Autodesk Inventor part; units mm, degrees
ref_plane "YZ Plane" through (0, 0, 0) normal (1, 0, 0) x (0, 1, 0)
ref_plane "XZ Plane" through (0, 0, 0) normal (0, 1, 0) x (-1, 0, 0)
ref_plane "XY Plane" through (0, 0, 0) normal (0, 0, 1) x (1, 0, 0)
sketch "Sketch1" plane through (0, 0, 0) normal (0, 1, 0) x (-1, 0, 0)
  line L0 (2.1258, 0) -> (-2.1258, 0) construction
  line L1 (0, 4.2515) -> (0, -4.2515) construction
  line L2 (20, 10) -> (-20, 10)
  line L3 (-20, 10) -> (-20, -10)
  line L4 (-20, -10) -> (20, -10)
  line L5 (20, -10) -> (20, 10)
  point P0 (0, 0)
  point P1 (0, 0)
  dimension "d1" = 20
  dimension "d2" = 20
  dimension "d3" = 20
extrude "Extrusion1" add sketch "Sketch1" along normal blind 7
sketch "Sketch2" plane through (0, 7, 0) normal (0, 1, 0) x (1, 0, 0)
  point P0 (0, 0)
  point P1 (10, 0)
  dimension "d6" = 10
hole "Hole1" at (10, 7, 0) direction (0, -1, 0) diameter 5.5 end through all countersink diameter 10.4 countersink angle 90
ref_plane "Work Plane1" through (0, 5, 0) normal (0, 1, 0) x (1, 0, 0)
sketch "Sketch3" plane through (0, 5, 0) normal (0, 1, 0) x (1, 0, 0)
  circle A0 centre (-8.9944, 0) radius 3
  point P0 (0, 0)
  dimension "d15" = 6
extrude "Extrusion2" cut sketch "Sketch3" against normal blind 1.7
fillet "Fillet1" radius 2 4 edges at (-20, 3.5, 10) (-20, 3.5, -10) (20, 3.5, 10) (20, 3.5, -10)
properties part number "MagnetHolderV1"
CAD build for the part. Positions are in the model's coordinates, mm. A direction names the side the tool comes from. Give positions to 0.01 mm unless a question says otherwise; leave off trailing zeros. Write each loop counter-clockwise with the first axis right and the second up, starting at its lowest first coordinate (ties: lowest second). Pieces come first, ordered by that corner, then holes. Notation, with made-up numbers: M -11.75,55 L 28.25,55 A23 cw 28.25,75 Z; hole C 61.25,-26.5 d3. An arc over 180 degrees is marked long. Put each result on its own line as item: value. Start each with the question number.
(1) Band-saw the part on D-D, the plane y = 4. Write the cut outline in (x, z), and give its area (3 significant figures).
(2) Flat gauge pin, fed straight in: pin 1 Ø12 at (x, z) = (-14.5, -4.5) entering from -Y. Where does the tip first touch, or does it go through?
(3) Band-saw the part on C-C, the plane y = 6.25. Write the cut outline in (x, z).
(4) Which spindle directions (+Z, -Z, +X, -X, +Y, -Y) get a long thin tool onto all of the face, cutting with end or side? Do faces 4 (the face through (-9, 3.3, 0)), 5 (the face through (0, 7, 0)). Say none if no direction does.
(5) Probe L1, parallel to X at y = 3.9, z = 0; L2, parallel to X at y = 2.85, z = 0; L3, parallel to X at y = 4.6, z = 0. List the from-to ranges inside material, lowest first.
(6) Band-saw the part on A-A, the plane z = 0. Write the cut outline in (x, y).
(7) Mould opens along Z. For faces 1 (the face through (20, 3, 0)), 2 (the face through (-6.223, 4.162, 1.149)), 3 (the face through (19.43, 3.55, -9.4)) say: +Z half, -Z half, draft (parallel to the pull), parting line (faces both ways), or undercut.
(8) Band-saw the part on B-B, the plane x = 10. Write the cut outline in (y, z), and give its area (3 significant figures).
Response values:
1. outline: M -20,-8 A2 ccw -18,-10 L 18,-10 A2 ccw 20,-8 L 20,8 A2 ccw 18,10 L -18,10 A2 ccw -20,8 Z; hole C -8.99,0 d6; hole C 10,0 d5.5
1. area: 745 mm2
2. pin 1: stops at y = 0
3. outline: M -20,-8 A2 ccw -18,-10 L 18,-10 A2 ccw 20,-8 L 20,8 A2 ccw 18,10 L -18,10 A2 ccw -20,8 Z; hole C 10,0 d8.9
4. face 4: none
4. face 5: +Z, -Z, +X, -X, +Y
5. L1: x = -20 to -11.99, -5.99 to 7.25, 12.75 to 20
5. L2: x = -20 to 7.25, 12.75 to 20
5. L3: x = -20 to -11.99, -5.99 to 7.2, 12.8 to 20
6. outline: M -20,0 L 7.25,0 L 7.25,4.55 L 4.8,7 L -20,7 Z; M 12.75,0 L 20,0 L 20,7 L 15.2,7 L 12.75,4.55 Z; hole M -11.99,3.3 L -5.99,3.3 L -5.99,5 L -11.99,5 Z
7. face 1: draft
7. face 2: undercut
7. face 3: -Z half
8. outline: M 0,-10 L 7,-10 L 7,-5.2 L 4.55,-2.75 L 0,-2.75 Z; M 0,2.75 L 4.55,2.75 L 7,5.2 L 7,10 L 0,10 Z
8. area: 95.5 mm2
